from build123d import *

# Parameters (mm, degrees)
SKETCH_1_R          = 7
EXTRUDE_1_DEPTH     = 1.5
CHAMFER_1_SIZE      = 1.2
CHAMFER_1_SIZE2     = 2.078460969
SKETCH_2_R          = 4.4
SKETCH_2_R_2        = 4.2
CUT_EXTRUDE_1_DEPTH = 1
SKETCH_3_R          = 6
EXTRUDE_2_DEPTH     = 21.5
FILLET_1_R          = 1


with BuildPart() as part:
    # 草图1 → 凸台-拉伸1 (new body)
    with BuildSketch(Plane.XY):
        Circle(SKETCH_1_R)
    extrude(amount=EXTRUDE_1_DEPTH)

    # 倒角1
    chamfer_1_edges = [part.edges().sort_by_distance(p)[0] for p in [
        (-7, 0, 1.5),
    ]]
    chamfer_1_side = [part.faces().sort_by_distance(p)[0] for p in [
        (-7, 0, 0.75),
    ]]
    chamfer(chamfer_1_edges, length=CHAMFER_1_SIZE, length2=CHAMFER_1_SIZE2, reference=chamfer_1_side[0])

    # 草图2 → 切除-拉伸1 (cut)
    # profile 1 of 3: a face of its own
    with BuildSketch(Plane.XY.offset(1.5)):
        Circle(SKETCH_2_R)
        Circle(SKETCH_2_R_2, mode=Mode.SUBTRACT)
    # profile 2 of 3: a face of its own
    with BuildSketch(Plane.XY.offset(1.5)):
        with BuildLine():
            Line((-1.606969024, 1.915111108), (-1.928362829, 2.298133329))
            ThreePointArc((-1.928362829, 2.298133329), (0, -3), (1.928362829, 2.298133329))
            Line((1.928362829, 2.298133329), (1.606969024, 1.915111108))
            ThreePointArc((1.606969024, 1.915111108), (0, -2.5), (-1.606969024, 1.915111108))
        make_face()
    # profile 3 of 3: a face of its own
    with BuildSketch(Plane.XY.offset(1.5)):
        Polygon((-0.3, 1.4), (0.3, 1.4), (0.3, 3.2), (0, 3.2), (-0.3, 3.2), align=None)
    extrude(amount=-CUT_EXTRUDE_1_DEPTH, mode=Mode.SUBTRACT)

    # 草图3 → 凸台-拉伸2 (add)
    with BuildSketch(Plane(origin=(0, 0, 0), x_dir=(-1, 0, 0), z_dir=(0, 0, -1))):
        with Locations(Location((0, 0, 0), (0, 0, 180))):
            Circle(SKETCH_3_R)
    extrude(amount=EXTRUDE_2_DEPTH)

    # 圆角1
    fillet_1_edges = [part.edges().sort_by_distance(p)[0] for p in [
        (-6, 0, -21.5),
    ]]
    fillet(fillet_1_edges, radius=FILLET_1_R)


solid = part.part
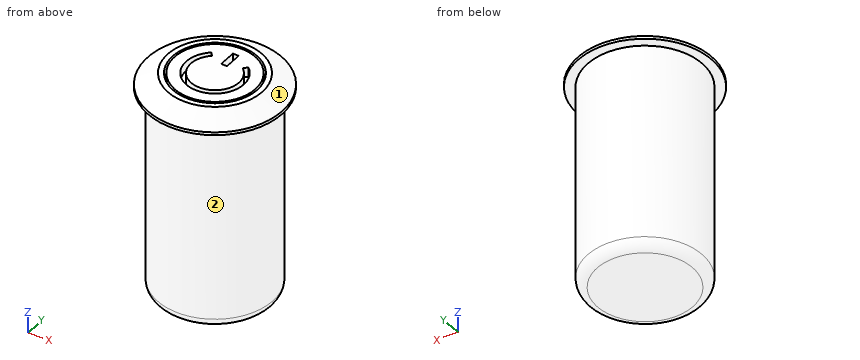
Geometry check sheet. Reference: the model listing, model coordinates, mm. Face numbers are marked on the shaded views. A direction names the side the tool comes from. Give positions to 0.01 mm unless a question says otherwise; leave off trailing zeros. Write each loop counter-clockwise with the first axis right and the second up, starting at its lowest first coordinate (ties: lowest second). Pieces come first, ordered by that corner, then holes. Notation, with made-up numbers: M -10.5,-36.75 L 32.5,-36.75 A26 ccw 32.5,-12.75 Z; hole C 77,35 d3. An arc over 180 degrees is marked long. Answer as CSV lines item,"result". Start each with the question number.
Q1. Go/stop test with flat-tipped pins: pin 1 (4 mm diameter, centred on x = -1.5, z = -3, fed in from -Y); pin 2 (1 mm diameter, centred on y = -3, z = -13.5, fed in from +X); pin 3 (0.7 mm diameter, centred on x = 0, z = 1, fed in from +Y). Record where each tip stops, or that it passes through.
Q2. Section check A-A, the plane x = 0. Record the cut outline in (y, z).
Q3. Material ranges on L1, parallel to Y at x = 0, z = 1.15; L2, parallel to Y at x = 0, z = 1.2; L3, parallel to X at y = -0.25, z = -6, recorded low to high.
Q4. Section check B-B, the plane y = 0. Record the cut outline in (x, z), then the cut area to 3 significant figures.
Q5. Tool access check on the marked faces 1 and 2. Record the directions out of +Z, -Z, +X, -X, +Y, -Y that give a thin tool (end or side, any length) a straight path to the whole face; none if there is none.
Q6. Section check C-C, the plane z = -5.25. Record the cut outline in (x, y).
Geometry says:
1,pin 1,"y = -6"
1,pin 2,"x = 5.45"
1,pin 3,"y = 6.39"
2,outline,"M -7,0 L -6,0 L -6,-20.5 A1 ccw -5,-21.5 L 5,-21.5 A1 ccw 6,-20.5 L 6,0 L 7,0 L 7,0.3 L 4.92,1.5 L 4.4,1.5 L 4.4,0.5 L 4.2,0.5 L 4.2,1.5 L 3.2,1.5 L 3.2,0.5 L 1.4,0.5 L 1.4,1.5 L -2.5,1.5 L -2.5,0.5 L -3,0.5 L -3,1.5 L -4.2,1.5 L -4.2,0.5 L -4.4,0.5 L -4.4,1.5 L -4.92,1.5 L -7,0.3 Z"
3,L1,"-5.53 to -4.4, -4.2 to -3, -2.5 to 1.4, 3.2 to 4.2, 4.4 to 5.53"
3,L2,"-5.44 to -4.4, -4.2 to -3, -2.5 to 1.4, 3.2 to 4.2, 4.4 to 5.44"
3,L3,"-5.99 to 5.99"
4,outline,"M -7,0 L -6,0 L -6,-20.5 A1 ccw -5,-21.5 L 5,-21.5 A1 ccw 6,-20.5 L 6,0 L 7,0 L 7,0.3 L 4.92,1.5 L 4.4,1.5 L 4.4,0.5 L 4.2,0.5 L 4.2,1.5 L 3,1.5 L 3,0.5 L 2.5,0.5 L 2.5,1.5 L -2.5,1.5 L -2.5,0.5 L -3,0.5 L -3,1.5 L -4.2,1.5 L -4.2,0.5 L -4.4,0.5 L -4.4,1.5 L -4.92,1.5 L -7,0.3 Z"
4,area,"275 mm^2"
5,face 1,"+Z"
5,face 2,"-Z"
6,outline,"C 0,0 d12"
